Part model, mm, in its own coordinate system. Face numbers are marked on the shaded views. A direction names the side the tool comes from. Coordinates: 2 decimals unless noted, no trailing zeros. Loops run counter-clockwise (first coordinate to the right, second up) from the corner with the lowest first, then second, coordinate; pieces in that order, holes last. Notation, with made-up numbers: M -7,29.5 L 31,29.5 A23 cw 31,49.5 Z; hole C 53,74.5 d3. An arc over 180 degrees is marked long. Use a Markdown table: item, result. Add a question column.
1) Wall check: probe 1 along Y at (x, z) = (5.5, 0); probe 2 along X at (y, z) = (0.5, 14); probe 3 along Z at (x, y) = (-98.5, 3). Give the ranges that are in metal, low to high. Write a range as from..to.
2) Tool access for the marked faces 1, 2 and 3: list every direction of +Z, -Z, +X, -X, +Y, -Y with a clear straight run to the whole face (end or side of a thin tool).
3) Band-saw the part on B-B (x = -23.5). List the corners of the cut face in (y, z), plus the area to 3 significant figures.
4) Pin check, flat tips, straight feed: pin 1 Ø2 at (x, z) = (-102.5, -8) entering from -Y; pin 2 Ø4 at (y, z) = (4, -12.5) entering from -X; pin 3 Ø12 at (x, y) = (-64.5, 2) entering from +Z. Stop position of each tip, or through.
5) Band-saw the part on A-A (x = -71). List the corners of the cut face in (y, z).
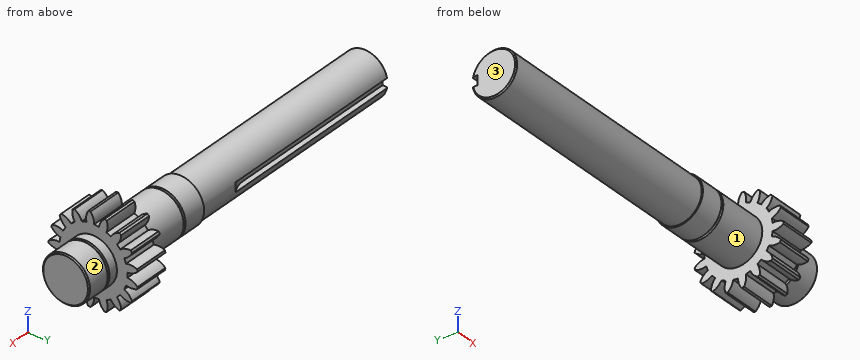
from build123d import *

# Parameters (mm, degrees)
BASPROSKE_W         = 15
BASPROSKE_H         = 19
TOOTHCUT_DEPTH      = 31.773365107
TEETHCUTS_COUNT     = 17
TEETHCUTS_ANGLE     = 338.823529412
BORSKE_R            = 0.4
BORE_DEPTH          = 50.0000508
SKETCH1_R           = 10
BOSS_EXTRUDE1_DEPTH = 15
BOSS_EXTRUDE2_START = 32
SKETCH2_R           = 10
BOSS_EXTRUDE2_DEPTH = 32
BOSS_EXTRUDE3_START = 32
SKETCH2_3_R         = 9.5
BOSS_EXTRUDE3_DEPTH = 100
CUT_EXTRUDE1_DEPTH  = 2
SKETCH4_W           = 1
SKETCH4_H           = 1
CHAMFER1_SIZE       = 0.5


with BuildPart() as part:
    # BasProSke → Base-Revolve (revolve)
    with BuildSketch(Plane(origin=(0, 0, 0), x_dir=(1, 0, 0), z_dir=(0, 1, 0)), mode=Mode.PRIVATE) as base_revolve_sk:
        with Locations((7.5, 9.5)):
            Rectangle(BASPROSKE_W, BASPROSKE_H)
    revolve(base_revolve_sk.sketch.rotate(Axis((-10, 0, 0), (1, 0, 0)), 180), axis=Axis((-10, 0, 0), (1, 0, 0)))

    # TooCutSke → ToothCut (cut, through all)
    with BuildSketch(Plane(origin=(0, 0, 0), x_dir=(0, 0, -1), z_dir=(1, 0, 0))):
        with BuildLine():
            ThreePointArc((1.020352389, 14.463052306), (0, 14.499), (-1.020352389, 14.463052306))
            ThreePointArc((-1.020352389, 14.463052306), (-1.632621885, 16.804485203), (-3.026143023, 18.783192049))
            ThreePointArc((-3.026143023, 18.783192049), (0, 19.0254), (3.026143023, 18.783192049))
            ThreePointArc((3.026143023, 18.783192049), (1.632621885, 16.804485203), (1.020352389, 14.463052306))
        make_face()
    toothcut = extrude(amount=TOOTHCUT_DEPTH, mode=Mode.SUBTRACT)

    # TeethCuts: ToothCut ×17 about axis
    teethcuts_axis = Axis((-10, 0, 0), (1, 0, 0))
    for i in range(1, TEETHCUTS_COUNT):
        add(toothcut.rotate(teethcuts_axis, i * TEETHCUTS_ANGLE / (TEETHCUTS_COUNT - 1)), mode=Mode.SUBTRACT)

    # BorSke → Bore (cut, symmetric)
    with BuildSketch(Plane(origin=(0, 0, 0), x_dir=(0, 0, -1), z_dir=(1, 0, 0))):
        with Locations(Location((0, 0, 0), (0, 0, 180))):
            Circle(BORSKE_R)
    extrude(amount=BORE_DEPTH, both=True, mode=Mode.SUBTRACT)

    # Sketch1 → Boss-Extrude1 (add)
    with BuildSketch(Plane(origin=(15, 0, 0), x_dir=(0, 0, -1), z_dir=(1, 0, 0))):
        with Locations(Location((0, 0, 0), (0, 0, 180))):
            Circle(SKETCH1_R)
    extrude(amount=BOSS_EXTRUDE1_DEPTH)

    # Sketch2 → Boss-Extrude2 (add)
    with BuildSketch(Plane.ZY.offset(BOSS_EXTRUDE2_START)):
        Circle(SKETCH2_R)
    extrude(amount=-BOSS_EXTRUDE2_DEPTH)

    # Sketch2<3> → Boss-Extrude3 (add)
    with BuildSketch(Plane.ZY.offset(BOSS_EXTRUDE3_START)):
        Circle(SKETCH2_3_R)
    extrude(amount=BOSS_EXTRUDE3_DEPTH)

    # Sketch3 → Cut-Extrude1 (cut, symmetric)
    with BuildSketch(Plane.XY):
        with BuildLine():
            Line((-132, 9.5), (-132, 7))
            Line((-132, 7), (-57, 7))
            ThreePointArc((-57, 7), (-53.127016654, 7.642183308), (-49.668560851, 9.5))
            Line((-49.668560851, 9.5), (-132, 9.5))
        make_face()
    extrude(amount=CUT_EXTRUDE1_DEPTH, both=True, mode=Mode.SUBTRACT)

    # Sketch4 → Cut-Revolve1 (revolve, cut)
    with BuildSketch(Plane.XY, mode=Mode.PRIVATE) as cut_revolve1_sk:
        with Locations((19.5, 9.5)):
            Rectangle(SKETCH4_W, SKETCH4_H)
        with Locations((-21.5, 9.5)):
            Rectangle(SKETCH4_W, SKETCH4_H)
    revolve(cut_revolve1_sk.sketch.rotate(Axis((0, 0, 0), (-1, 0, 0)), 90), axis=Axis((0, 0, 0), (-1, 0, 0)), mode=Mode.SUBTRACT)

    # Chamfer1
    chamfer1_edges = [part.edges().sort_by_distance(p)[0] for p in [
        (30, 0, -10),
        (-132, -7.39087275, -5.968668193),
    ]]
    chamfer(chamfer1_edges, length=CHAMFER1_SIZE)


solid = part.part
Entries:
| question | item | result |
|---|---|---|
| 1 | probe 1 | -19..-0.4, 0.4..14.5 |
| 1 | probe 2 | 0..15 |
| 1 | probe 3 | -9.01..9.01 |
| 2 | face 1 | -X |
| 2 | face 2 | +X |
| 2 | face 3 | +Z, -Z, -X, +Y, -Y |
| 3 | outline | C 0,0 d20 |
| 3 | area | 314 mm2 |
| 4 | pin 1 | y = -6.42 |
| 4 | pin 2 | x = 0 |
| 4 | pin 3 | z = 9.5 |
| 5 | outline | M 7,-2 L 7,2 L 9.29,2 A9.5 ccw long 9.29,-2 Z |
